Autodesk Inventor part; units mm, degrees
ref_plane "YZ Plane" through (0, 0, 0) normal (1, 0, 0) x (0, 1, 0)
ref_plane "XZ Plane" through (0, 0, 0) normal (0, 1, 0) x (-1, 0, 0)
ref_plane "XY Plane" through (0, 0, 0) normal (0, 0, 1) x (1, 0, 0)
sketch "Sketch1" plane through (0, 0, 0) normal (1, 0, 0) x (0, 1, 0)
  line L0 (-50, -18) -> (50, -18)
  line L1 (50, -18) -> (50, 18)
  line L2 (50, 18) -> (-50, 18)
  line L3 (-50, 18) -> (-50, -18)
  line L4 (-50, -18) -> (50, 18) construction
  line L5 (50, -18) -> (-50, 18) construction
  point P0 (0, 0)
  dimension "d0" = 36
  dimension "d1" = 100
extrude "Extrusion1" add sketch "Sketch1" along normal blind 3
sketch "Sketch2" plane through (0, 0, 0) normal (-1, 0, 0) x (0, 0, 1)
  line L0 (-5, -22) -> (5, -22)
  line L1 (5, -22) -> (5, -25)
  line L2 (5, -25) -> (-5, -25)
  line L3 (-5, -25) -> (-5, -22)
  line L4 (18, -50) -> (-18, -50)
  point P0 (0, 0)
  point P1 (0, -22)
  dimension "d4" = 10
  dimension "d5" = 3
  dimension "d6" = 25
extrude "Extrusion2" cut sketch "Sketch2" against normal blind 3
sketch "Sketch3" plane through (0, 0, 0) normal (-1, 0, 0) x (0, 0, 1)
  line L0 (-18, -50) -> (-8, -50)
  line L1 (-8, -50) -> (-8, -53)
  line L2 (-8, -53) -> (-18, -53)
  line L3 (-18, -53) -> (-18, -50)
  line L4 (18, -50) -> (8, -50)
  line L5 (8, -50) -> (8, -53)
  line L6 (8, -53) -> (18, -53)
  line L7 (18, -53) -> (18, -50)
  point P0 (0, 0)
  dimension "d9" = 10
  dimension "d10" = 3
  dimension "d11" = 10
  dimension "d12" = 3
extrude "Extrusion3" add sketch "Sketch3" against normal blind 3
properties part number "Back support"
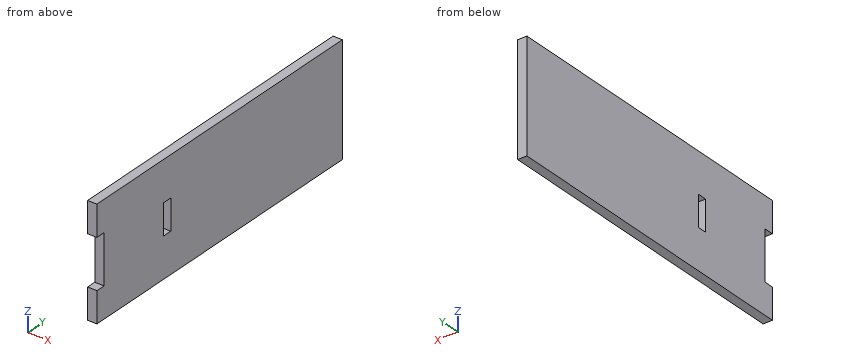
Model file for the job. Use its own axes, mm. Round coordinates to 2 decimals unless told otherwise and drop trailing zeros. Loops run counter-clockwise (first coordinate to the right, second up) from the corner with the lowest first, then second, coordinate; pieces in that order, holes last.
1. Band-saw the part on A-A, the plane x = 1.5. List the corners of the cut face in (y, z).
Check values:
outline: (-53, -18) - (50, -18) - (50, 18) - (-53, 18) - (-53, 8) - (-50, 8) - (-50, -8) - (-53, -8) - close; hole (-25, -5) - (-22, -5) - (-22, 5) - (-25, 5) - close
2. Band-saw the part on B-B, the plane z = -2.5. List the corners of the cut face in (x, y).
Check values:
outline: (0, -50) - (3, -50) - (3, -25) - (0, -25) - close; (0, -22) - (3, -22) - (3, 50) - (0, 50) - close
3. Wall check: probe 1 along Y at (x, z) = (1.05, 0.5); probe 2 along Y at (x, z) = (0.9, -7). Give the ranges that are in metal, low to high.
Check values:
probe 1: y = -50 to -25, -22 to 50
probe 2: y = -50 to 50
4. Drop a flat-ended pin along its axis: P1, Ø1.5, axis at x = 1.5, z = 0.5, coming from the -Y side. Give the stop position or say it passes through.
Check values:
P1: stops at y = -50
